Check sheet for the modelled part. Datum: model origin and axes. Units: mm. Give positions to 0.01 mm unless a question says otherwise; leave off trailing zeros. Loops run counter-clockwise (first coordinate to the right, second up) from the corner with the lowest first, then second, coordinate; pieces in that order, holes last. Notation, with made-up numbers: (-40, 46.5) - (6, 46.5) arc R28 cw to (6, 69.5) - close; hole circle Ø7 at (44.5, 54.5). An arc over 180 degrees is marked (long way). Use CSV: the item, a comma, the result in double quotes.
Autodesk Inventor part; units mm, degrees
ref_plane "YZ Plane" through (0, 0, 0) normal (1, 0, 0) x (0, 1, 0)
ref_plane "XZ Plane" through (0, 0, 0) normal (0, 1, 0) x (-1, 0, 0)
ref_plane "XY Plane" through (0, 0, 0) normal (0, 0, 1) x (1, 0, 0)
sketch "Sketch1" plane through (0, 0, 0) normal (0, 1, 0) x (-1, 0, 0)
  line L0 (7.1803, 16.0154) -> (7.1803, -27.9846)
  line L1 (6.6803, -28.4846) -> (0.2201, -28.4846)
  line L2 (-0.2762, -27.9236) -> (5.1264, 16.0764)
  line L3 (5.6226, 16.5154) -> (6.6803, 16.5154)
  arc A0 (6.6803, -28.4846) -> (7.1803, -27.9846) centre (6.6803, -27.9846) ccw
  arc A1 (-0.2762, -27.9236) -> (0.2201, -28.4846) centre (0.2201, -27.9846) ccw
  arc A2 (7.1803, 16.0154) -> (6.6803, 16.5154) centre (6.6803, 16.0154) ccw
  arc A3 (5.6226, 16.5154) -> (5.1264, 16.0764) centre (5.6226, 16.0154) ccw
  point P0 (0, 0)
  point P1 (7.1803, 16.5154)
  point P2 (7.1803, -28.4846)
  point P3 (5.1803, 16.5154)
  dimension "d0" = 45
  dimension "d1" = 7
  dimension "d2" = 2
  dimension "d3" = 0.5
  dimension "d4" = 0.5
  dimension "d5" = 0.5
extrude "Extrusion1" add sketch "Sketch1" along normal blind 7
properties part number "Wedge - V2"
1. Sectioned sample at B-B, the plane x = -4. Record the boundary of the cut face in (y, z), and give its area (3 significant figures).
Completed:
outline,"(0, -28.48) - (7, -28.48) - (7, 6.9) - (0, 6.9) - close"
area,"248 mm²"
2. Go/stop test with a flat-tipped pin: pin 1 Ø2 at (y, z) = (5, 4) entering from +X. Record where the tip stops, or that it passes through.
Completed:
pin 1,"stops at x = -3.52"
3. Sectioned sample at A-A, the plane y = 4.5. Record the boundary of the cut face in (x, z), and give its area (3 significant figures).
Completed:
outline,"(-7.18, -27.98) arc R0.5 ccw to (-6.68, -28.48) - (-0.22, -28.48) arc R0.5 ccw to (0.28, -27.92) - (-5.13, 16.08) arc R0.5 ccw to (-5.62, 16.52) - (-6.68, 16.52) arc R0.5 ccw to (-7.18, 16.02) - close"
area,"214 mm²"
4. Scan lines: line 1 along X through (y, z) = (6.25, 12.5); line 2 along X through (y, z) = (4, -12.5). Record each from-to range of solid material in increasing order.
Completed:
line 1,"x = -7.18 to -4.69"
line 2,"x = -7.18 to -1.62"
5. Sectioned sample at C-C, the plane z = -5. Record the boundary of the cut face in (x, y).
Completed:
outline,"(-7.18, 0) - (-2.54, 0) - (-2.54, 7) - (-7.18, 7) - close"
